Can you work these out from the model? Positions are in its coordinate system, mm. A direction names the side the tool comes from. Give positions to 0.01 mm unless a question says otherwise; leave off trailing zeros. Order: outer loops, then holes, each group sorted by start corner. A loop starts at its lowest first (then second) coordinate and runs counter-clockwise, first axis right, second up. Notation, with made-up numbers: M 84,12.5 L 99,12.5 A23 ccw 99,33.5 Z; hole C -28.75,5.5 d6. An arc over 180 degrees is marked long. Write each question's results on one line, items separated by ' | '.
from build123d import *

# Parameters (mm, degrees)
SKETCH_1_R          = 11
EXTRUDE_1_DEPTH     = 12
SKETCH_2_R          = 2.75
CUT_EXTRUDE_1_DEPTH = 39.356876828


with BuildPart() as part:
    # 草图1 → 凸台-拉伸1 (new body)
    with BuildSketch(Plane.XY):
        with BuildLine():
            Line((14.5, 10), (25.5, 10))
            ThreePointArc((25.5, 10), (26.207106781, 9.707106781), (26.5, 9))
            Line((26.5, 9), (26.5, 0))
            Line((26.5, 0), (-26.5, 0))
            Line((-26.5, 0), (-26.5, 9))
            ThreePointArc((-26.5, 9), (-26.207106781, 9.707106781), (-25.5, 10))
            Line((-25.5, 10), (-14.5, 10))
            Line((-14.5, 10), (-14.5, 24))
            ThreePointArc((-14.5, 24), (-11.278174593, 31.778174593), (-3.5, 35))
            Line((-3.5, 35), (3.5, 35))
            ThreePointArc((3.5, 35), (11.278174593, 31.778174593), (14.5, 24))
            Line((14.5, 24), (14.5, 10))
        make_face()
        with Locations((0, 20)):
            Circle(SKETCH_1_R, mode=Mode.SUBTRACT)
    extrude(amount=EXTRUDE_1_DEPTH)

    # 草图2 → 切除-拉伸1 (cut, through all)
    with BuildSketch(Plane(origin=(0, 10, 0), x_dir=(1, 0, 0), z_dir=(0, 1, 0))):
        with Locations(Location((-20.5, -6, 0), (0, 0, 180))):
            Circle(SKETCH_2_R)
        with Locations((20.5, -6)):
            Circle(SKETCH_2_R)
    extrude(amount=-CUT_EXTRUDE_1_DEPTH, mode=Mode.SUBTRACT)


solid = part.part
(1) Imagine slicing it at A-A, the plane z = 6. Write out the boundary of the cut face in (x, y).
Data:
outline: M -26.5,0 L -23.25,0 L -23.25,10 L -25.5,10 A1 ccw -26.5,9 Z; M -17.75,0 L 17.75,0 L 17.75,10 L 14.5,10 L 14.5,24 A11 ccw 3.5,35 L -3.5,35 A11 ccw -14.5,24 L -14.5,10 L -17.75,10 Z; M 23.25,0 L 26.5,0 L 26.5,9 A1 ccw 25.5,10 L 23.25,10 Z; hole C 0,20 d22
(2) We'd pull the mould along X, two halves only. Please class faces 3 (the face through (-17.6, 10, 5.9)), 4 (the face through (-14.5, 17, 6)), 5 (the face through (-2.38, 9.26, 5.92)): +X half, -X half, draft (parallel to the pull), parting line (faces both ways), or undercut.
Data:
face 3: draft | face 4: -X half | face 5: undercut
(3) I need wall thicknesses on L1, parallel to X at y = 8.5, z = 8.25; L2, parallel to Y at x = 24, z = 11; L3, parallel to X at y = 5, z = 5. Which ranges of each line are inside material? Lowest first, please. Write a range as from..to.
Data:
L1: x = -26.5..-22.08, -18.92..18.92, 22.08..26.5 | L2: y = 0..10 | L3: x = -26.5..-23.06, -17.94..17.94, 23.06..26.5
(4) Will these pins go through, and if not, where does the flat tip stop? P1, Ø1.5, axis at y = 15, z = 7.5, coming from the -X side; P2, Ø4, axis at x = 13, z = 6.5, coming from the +Y side; P3, Ø6, axis at y = 18, z = 4.5, coming from the +X side.
Data:
P1: stops at x = -14.5 | P2: stops at y = 32.05 | P3: stops at x = 14.5
(5) Imagine slicing it at C-C, the plane y = 19. Write out the boundary of the cut face in (x, z).
Data:
outline: M -14.5,0 L -10.95,0 L -10.95,12 L -14.5,12 Z; M 10.95,0 L 14.5,0 L 14.5,12 L 10.95,12 Z
(6) For faces 1 (the face through (6, 10, 0)), 2 (the face through (17, 10, 6)), which set-ups out of +Z, -Z, +X, -X, +Y, -Y let a thin tool reach every point of the face, with its end or its side?
Data:
face 1: -Z, +X, -X, +Y, -Y | face 2: +Z, -Z, +X, +Y
(7) Imagine slicing it at B-B, the plane x = 0. Write out the boundary of the cut face in (y, z), plus the area to 3 significant figures.
Data:
outline: M 0,0 L 9,0 L 9,12 L 0,12 Z; M 31,0 L 35,0 L 35,12 L 31,12 Z | area: 156 mm2
